CAD build for the part. Positions are in the model's coordinates, mm. A direction names the side the tool comes from. Coordinates: 2 decimals unless noted, no trailing zeros. Return JSON: item names as keys, results as strings.
Autodesk Inventor part; units mm, degrees
ref_plane "YZ Plane" through (0, 0, 0) normal (1, 0, 0) x (0, 1, 0)
ref_plane "XZ Plane" through (0, 0, 0) normal (0, 1, 0) x (-1, 0, 0)
ref_plane "XY Plane" through (0, 0, 0) normal (0, 0, 1) x (1, 0, 0)
sketch "Эскиз1" plane through (0, 0, 0) normal (0, 0, 1) x (1, 0, 0)
  line L0 (-21.25, 15.93) -> (21.25, 15.93)
  line L1 (-16.25, 17.93) -> (-18.25, 15.93)
  line L2 (-16.25, 17.93) -> (16.25, 17.93)
  line L3 (16.25, 17.93) -> (18.25, 15.93)
  line L4 (-26.02, 3) -> (26.02, 3)
  line L5 (-21.25, 15.93) -> (-21.25, 5)
  line L6 (30, 22.93) -> (-30, 22.93)
  line L7 (-25.52, 22.93) -> (-25.52, 3)
  line L8 (-18.25, 15.93) -> (-18.75, 15.93)
  line L9 (0, 17.93) -> (0, 19.43)
  line L10 (-18.75, 15.93) -> (-14.5074, 15.93) construction
  line L11 (-21.25, 15.93) -> (-21.25, 22.93)
  line L12 (-21.25, 22.93) -> (0, 22.93)
  line L13 (0, 17.93) -> (0, 22.93)
  line L14 (-21.25, 15.98) -> (21.25, 15.98)
  line L15 (-18.75, 15.93) -> (-11.809, 15.93) construction
  line L16 (0, 19.43) -> (-15.25, 19.43)
  line L17 (-15.25, 19.43) -> (-18.75, 15.93)
  line L18 (-15.25, 19.43) -> (-18.75, 19.43)
  line L19 (-18.75, 19.43) -> (-18.75, 15.93)
  line L20 (21.25, 15.98) -> (21.25, 22.93)
  line L21 (0, 22.93) -> (21.25, 22.93)
  line L22 (21.75, 21.33) -> (21.75, 22.93)
  line L23 (22.25, 21.33) -> (21.25, 21.33)
  line L24 (23.25, 22.93) -> (21.25, 19.73)
  spline S0 degree 2 poles (23.25, 22.93) (21.0575, 22.6489) (21.25, 19.73) knots 0 0 0 1 1 1
  line L25 (23.25, 22.93) -> (21.25, 22.93)
  line L26 (23.25, 19.73) -> (21.25, 19.73)
  line L27 (22.25, 21.33) -> (21.25, 21.33)
  line L28 (21.75, 21.33) -> (21.75, 22.93)
  line L29 (23.25, 22.93) -> (21.25, 22.93)
  line L30 (23.25, 22.93) -> (21.25, 19.73)
  spline S1 degree 2 poles (23.25, 22.93) (21.0575, 22.6489) (21.25, 19.73) knots 0 0 0 1 1 1
  line L31 (0, 17.93) -> (-3, 17.93)
  line L32 (-3, 17.93) -> (-4.5, 19.43)
  point P0 (-18.7, 15.98)
  point P1 (-18.75, 15.98)
  point P2 (21.75, 22.13)
  point P3 (22.7031, 19.73)
  point P4 (21.75, 22.13)
  point P5 (21.25, 20.6035)
  dimension "d0" = 0.5
  dimension "d1" = 1.5
  dimension "d3" = 0.05
  dimension "d28" = 3
revolve "Вращение1" add sketch "Эскиз1" angle 360 about axis through (0, 17.93, 0) along (0, 1, 0) contours L11 L6 L13 L16 L18 L19 L14 | L16 L9 L2 L32 | L6 L22 S0 L23 L20 | L6 S0 L22 | L23 S0 L20
sketch "Эскиз3" plane through (0, 22.93, 0) normal (0, 1, 0) x (1, 0, 0)
  circle A0 centre (0, 0) radius 1.7
  line L0 (0, 0) -> (0, 12)
  circle A1 centre (0, 0) radius 21.25
  circle A2 centre (0, 0) radius 15.75
  circle A3 centre (0, 12) radius 1.7
  circle A4 centre (-10.3923, 6) radius 1.7
  circle A5 centre (-10.3923, -6) radius 1.7
  circle A6 centre (0, -12) radius 1.7
  circle A7 centre (10.3923, -6) radius 1.7
  circle A8 centre (10.3923, 6) radius 1.7
  point P0 (-21.25, 0)
  dimension "d7" = 3.4
  dimension "d8" = 12
  dimension "d9" = 3.4
  dimension "d12" = 360
extrude "Выдавливание1" cut sketch "Эскиз3" against normal blind 10 contours A3 | A4 | A5 | A6 | A7 | A8
sketch "Эскиз4" plane through (0, 22.93, 0) normal (0, 1, 0) x (1, 0, 0)
  line L0 (0, 0) -> (0, 2.85)
  circle A0 centre (0, 12) radius 1.7
  line L1 (0, 12) -> (0, 9.15)
  line L2 (1.6454, 2.85) -> (3.2909, 0)
  line L3 (3.2909, 0) -> (1.6454, -2.85)
  line L4 (1.6454, -2.85) -> (-1.6454, -2.85)
  line L5 (-1.6454, -2.85) -> (-3.2909, 0)
  line L6 (-3.2909, 0) -> (-1.6454, 2.85)
  line L7 (-1.6454, 2.85) -> (1.6454, 2.85)
  line L8 (-1.6454, 9.15) -> (-3.2909, 12)
  line L9 (-3.2909, 12) -> (-1.6454, 14.85)
  line L10 (-1.6454, 14.85) -> (1.6454, 14.85)
  line L11 (1.6454, 14.85) -> (3.2909, 12)
  line L12 (3.2909, 12) -> (1.6454, 9.15)
  line L13 (1.6454, 9.15) -> (-1.6454, 9.15)
  line L14 (8.7469, 3.15) -> (7.1014, 6)
  line L15 (10.3923, 6) -> (7.9241, 4.575)
  line L16 (12.0378, 3.15) -> (8.7469, 3.15)
  line L17 (13.6832, 6) -> (12.0378, 3.15)
  line L18 (12.0378, 8.85) -> (13.6832, 6)
  line L19 (8.7469, 8.85) -> (12.0378, 8.85)
  line L20 (7.1014, 6) -> (8.7469, 8.85)
  line L21 (7.1014, -6) -> (8.7469, -3.15)
  line L22 (10.3923, -6) -> (7.9241, -4.575)
  line L23 (8.7469, -8.85) -> (7.1014, -6)
  line L24 (12.0378, -8.85) -> (8.7469, -8.85)
  line L25 (13.6832, -6) -> (12.0378, -8.85)
  line L26 (12.0378, -3.15) -> (13.6832, -6)
  line L27 (8.7469, -3.15) -> (12.0378, -3.15)
  line L28 (-1.6454, -9.15) -> (1.6454, -9.15)
  line L29 (0, -12) -> (0, -9.15)
  line L30 (-3.2909, -12) -> (-1.6454, -9.15)
  line L31 (-1.6454, -14.85) -> (-3.2909, -12)
  line L32 (1.6454, -14.85) -> (-1.6454, -14.85)
  line L33 (3.2909, -12) -> (1.6454, -14.85)
  line L34 (1.6454, -9.15) -> (3.2909, -12)
  line L35 (-8.7469, -3.15) -> (-7.1014, -6)
  line L36 (-10.3923, -6) -> (-7.9241, -4.575)
  line L37 (-12.0378, -3.15) -> (-8.7469, -3.15)
  line L38 (-13.6832, -6) -> (-12.0378, -3.15)
  line L39 (-12.0378, -8.85) -> (-13.6832, -6)
  line L40 (-8.7469, -8.85) -> (-12.0378, -8.85)
  line L41 (-7.1014, -6) -> (-8.7469, -8.85)
  line L42 (-7.1014, 6) -> (-8.7469, 3.15)
  line L43 (-10.3923, 6) -> (-7.9241, 4.575)
  line L44 (-8.7469, 8.85) -> (-7.1014, 6)
  line L45 (-12.0378, 8.85) -> (-8.7469, 8.85)
  line L46 (-13.6832, 6) -> (-12.0378, 8.85)
  line L47 (-12.0378, 3.15) -> (-13.6832, 6)
  line L48 (-8.7469, 3.15) -> (-12.0378, 3.15)
  dimension "d16" = 2.85
  dimension "d17" = 2.85
  dimension "d20" = 360
chamfer "Фаска1" distance 2 angle 45 6 edges at (-12.0923, 22.93, -6) (-12.0923, 22.93, 6) (-1.7, 22.93, -12) (8.6923, 22.93, -6) (8.6923, 22.93, 6) (-1.7, 22.93, 12)
properties part number "tire_cap2"
Item 1: Wall check: L1, parallel to Z at x = -1, y = 22.5; L2, parallel to Y at x = -11, z = 15; L3, parallel to X at y = 20.4, z = 6. Give the ranges that are in metal, low to high. Write a range as [from, to].
Findings below:
{"L1": "z = [-22.09, -15.11], [-8.89, 8.89], [15.11, 22.09]", "L2": "y = [19.43, 22.93]", "L3": "x = [-20.39, -12.09], [-8.69, 8.69], [12.09, 20.39]"}
Item 2: Band-saw the part on A-A, the plane x = 0. Count the separate pieces of the cut face and the enclosed holes in it, then the cut area to 3 significant figures.
Findings below:
{"separate pieces": "3", "enclosed holes": "0", "area": "148 mm²"}
Item 3: Drop flat-ended pins along their axis: P1, Ø3, axis at y = 17, z = -11.5, coming from the -X side; P2, Ø4, axis at x = -10, y = 17, coming from the -Z side; P3, Ø1, axis at y = 19.5, z = 18.5, coming from the -X side. Give the stop position or say it passes through.
Findings below:
{"P1": "stops at x = -18.75", "P2": "stops at z = -19.69", "P3": "stops at x = -11.29"}
Item 4: Which spindle directions (+Z, -Z, +X, -X, +Y, -Y) get a long thin tool onto all of the face, cutting with end or side? Do faces 4 (the cylindrical face through (-0.221, 20.19, -13.686)), 5 (the flat face through (-4, 19.43, -4)). Say none if no direction does.
Findings below:
{"face 4": "+Y, -Y", "face 5": "-Y"}
Item 5: Mould opens along X. For faces 1 (the flat face through (0, 15.98, -19)), 2 (the cylindrical face through (16.863, 18.324, -12.93)), 3 (the flat face through (0, 17.93, 0)) say: released by +X, released by -X, zero draft, split by the parting line, or undercut.
Findings below:
{"face 1": "zero draft", "face 2": "split by the parting line", "face 3": "undercut"}
